from build123d import *

# Parameters (mm, degrees)
SKETCH_1_W          = 82
SKETCH_1_H          = 66
SKETCH_1_R          = 1.6
SKETCH_1_R_2        = 1.35
EXTRUDE_1_DEPTH     = 2
FILLET_1_R          = 3
CUT_EXTRUDE_1_DEPTH = 10
SKETCH_3_R          = 27.5
SKETCH_3_R_2        = 24.5
SKETCH_3_W          = 10
SKETCH_3_H          = 3
EXTRUDE_1_2_DEPTH   = 2
SKETCH_4_R          = 1.1
CUT_EXTRUDE_2_DEPTH = 2
FILLET_2_R          = 1


with BuildPart() as part:
    # 草图1 → Extrude 1 (new body)
    with BuildSketch(Plane(origin=(0, 0, 0), x_dir=(1, 0, 0), z_dir=(0, 1, 0))):
        Rectangle(SKETCH_1_W, SKETCH_1_H)
        with Locations(Location((10, -30, 0), (0, 0, 270))):
            Circle(SKETCH_1_R, mode=Mode.SUBTRACT)
        with Locations(Location((-10, -30, 0), (0, 0, 270))):
            Circle(SKETCH_1_R, mode=Mode.SUBTRACT)
        with Locations(Location((-10, 30, 0), (0, 0, 270))):
            Circle(SKETCH_1_R, mode=Mode.SUBTRACT)
        with Locations(Location((10, 30, 0), (0, 0, 270))):
            Circle(SKETCH_1_R, mode=Mode.SUBTRACT)
        with Locations(Location((36, -27, 0), (0, 0, 270))):
            Circle(SKETCH_1_R_2, mode=Mode.SUBTRACT)
        with Locations(Location((36, 27, 0), (0, 0, 270))):
            Circle(SKETCH_1_R_2, mode=Mode.SUBTRACT)
        with Locations(Location((-36, 27, 0), (0, 0, 270))):
            Circle(SKETCH_1_R_2, mode=Mode.SUBTRACT)
        with Locations(Location((-36, -27, 0), (0, 0, 270))):
            Circle(SKETCH_1_R_2, mode=Mode.SUBTRACT)
    extrude(amount=EXTRUDE_1_DEPTH)

    # 圆角1
    fillet_1_edges = [part.edges().sort_by_distance(p)[0] for p in [
        (41, 1, 33),
        (-41, 1, 33),
        (-41, 1, -33),
        (41, 1, -33),
    ]]
    fillet(fillet_1_edges, radius=FILLET_1_R)

    # 草图2 → 切除-拉伸1 (cut)
    with BuildSketch(Plane(origin=(0, 2, 0), x_dir=(1, 0, 0), z_dir=(0, 1, 0))):
        with BuildLine():
            Line((32.385791926, 26), (-32.385791926, 26))
            ThreePointArc((-32.385791926, 26), (-33.729262234, 24.015665903), (-36, 23.25))
            Line((-36, 23.25), (-36, -23.25))
            ThreePointArc((-36, -23.25), (-33.729262234, -24.015665903), (-32.385791926, -26))
            Line((-32.385791926, -26), (32.385791926, -26))
            ThreePointArc((32.385791926, -26), (33.729262234, -24.015665903), (36, -23.25))
            Line((36, -23.25), (36, 23.25))
            ThreePointArc((36, 23.25), (33.729262234, 24.015665903), (32.385791926, 26))
        make_face()
    extrude(amount=-CUT_EXTRUDE_1_DEPTH, mode=Mode.SUBTRACT)

    # 草图3 → Extrude 1 2 (add)
    # profile 1 of 5: a face of its own
    with BuildSketch(Plane(origin=(0, 2, 0), x_dir=(1, 0, 0), z_dir=(0, 1, 0))):
        Circle(SKETCH_3_R)
        Circle(SKETCH_3_R_2, mode=Mode.SUBTRACT)
    # profile 2 of 5: a face of its own
    with BuildSketch(Plane(origin=(0, 2, 0), x_dir=(1, 0, 0), z_dir=(0, 1, 0))):
        Polygon((36.9, -25.8), (-35.1, 28.2), (-36.9, 25.8), (35.1, -28.2), align=None)
    # profile 3 of 5: a face of its own
    with BuildSketch(Plane(origin=(0, 2, 0), x_dir=(1, 0, 0), z_dir=(0, 1, 0))):
        Polygon((-35.1, -28.2), (36.9, 25.8), (35.1, 28.2), (-36.9, -25.8), align=None)
    # profile 4 of 5: a face of its own
    with BuildSketch(Plane(origin=(0, 2, 0), x_dir=(1, 0, 0), z_dir=(0, 1, 0))):
        with Locations((-31, 0)):
            Rectangle(SKETCH_3_W, SKETCH_3_H)
    # profile 5 of 5: a face of its own
    with BuildSketch(Plane(origin=(0, 2, 0), x_dir=(1, 0, 0), z_dir=(0, 1, 0))):
        with Locations((31, 0)):
            Rectangle(SKETCH_3_W, SKETCH_3_H)
    extrude(amount=-EXTRUDE_1_2_DEPTH)

    # 草图4 → 切除-拉伸2 (cut)
    with BuildSketch(Plane(origin=(0, 2, 0), x_dir=(1, 0, 0), z_dir=(0, 1, 0))):
        with Locations((36, 27)):
            Circle(SKETCH_4_R)
        with Locations((-36, 27)):
            Circle(SKETCH_4_R)
        with Locations((-36, -27)):
            Circle(SKETCH_4_R)
        with Locations((36, -27)):
            Circle(SKETCH_4_R)
    extrude(amount=-CUT_EXTRUDE_2_DEPTH, mode=Mode.SUBTRACT)

    # 圆角2
    fillet_2_edges = [part.edges().sort_by_distance(p)[0] for p in [
        (-34.150454583, 1, 23.737840937),
        (-8.958236434, 1, 26),
        (8.958236434, 1, 26),
        (-32.166666667, 1, 26),
        (32.166666667, 1, 26),
        (34.150454583, 1, 23.737840937),
        (34.150454583, 1, -23.737840937),
        (-8.958236434, 1, -26),
        (8.958236434, 1, -26),
        (32.166666667, 1, -26),
        (-32.166666667, 1, -26),
        (-34.150454583, 1, -23.737840937),
        (21.067248348, 1, 17.675436261),
        (-21.067248348, 1, 17.675436261),
        (0, 1, -1.875),
        (-18.663230817, 1, -15.872423113),
        (20.463230817, 1, 13.472423113),
        (0, 1, 1.875),
        (-22.867248348, 1, -15.275436261),
        (-22.867248348, 1, 15.275436261),
        (-27.459060435, 1, 1.5),
        (-36, 1, 1.5),
        (-27.459060435, 1, -1.5),
        (-36, 1, -1.5),
        (-20.463230817, 1, -13.472423113),
        (-20.463230817, 1, 13.472423113),
        (18.663230817, 1, 15.872423113),
        (-2.5, 1, 0),
        (-18.663230817, 1, 15.872423113),
        (2.5, 1, 0),
        (20.463230817, 1, -13.472423113),
        (21.067248348, 1, -17.675436261),
        (-21.067248348, 1, -17.675436261),
        (18.663230817, 1, -15.872423113),
        (22.867248348, 1, -15.275436261),
        (36, 1, 1.5),
        (27.459060435, 1, -1.5),
        (36, 1, -1.5),
        (22.867248348, 1, 15.275436261),
        (27.459060435, 1, 1.5),
        (-36, 1, -23.25),
        (36, 1, -23.25),
        (36, 1, 23.25),
        (-36, 1, 23.25),
    ]]
    fillet(fillet_2_edges, radius=FILLET_2_R)


solid = part.part
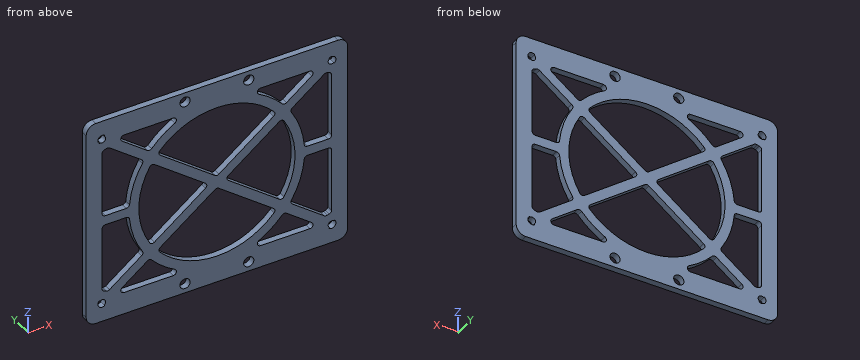
The listing builds one solid part. Answer for the finished solid, in the listing's coordinates (mm). Coordinates: 2 decimals unless noted, no trailing zeros. Order: outer loops, then holes, each group sorted by start corner. A loop starts at its lowest first (then second) coordinate and runs counter-clockwise, first axis right, second up. Notation, with made-up numbers: M -20,87 L -15,87 A35 ccw -15,119 Z; hole C 9,8 d4. An arc over 180 degrees is marked long. Use CSV: the item, a comma, the result in double quotes.
Q1. Section C-C (y = 1.65) is taken. Give the number of separate pieces and of enclosed holes in the cut face, then the cut area to 3 significant figures.
Here are the results:
separate pieces,"1"
enclosed holes,"20"
area,"2,620 mm2"
Q2. Straight lines are drawn through the part: L1, parallel to X at y = 1.35, z = -30; L2, parallel to X at y = 1.5, z = -27; L3, parallel to Z at x = 15, y = 0.2 (3 decimals). For each, find the intervals that lie inside material, in ascending order.
Here are the results:
L1,"-41 to -11.6, -8.4 to 8.4, 11.6 to 41"
L2,"-41 to -37.35, -34.9 to 34.9, 37.35 to 41"
L3,"-33 to -26, -23.049 to -19.371, -13.125 to -9.375, 9.375 to 13.125, 19.371 to 23.049, 26 to 33"
Q3. Given pin 1 Ø2.5 at (x, z) = (-10, -30) entering from +Y, flat-ended and moving along its own axis, determine where the tip first touches the part or whether it passes through.
Here are the results:
pin 1,"through"
Q4. Section A-A (x = -10) is taken. Determine the outline of the cut face in (y, z) (3 decimals), then the cut area to 3 significant figures.
Here are the results:
outline,"M 0,-33 L 2,-33 L 2,-31.6 L 0,-31.6 Z; M 0,-28.4 L 2,-28.4 L 2,-22.366 L 0,-22.366 Z; M 0,-9.375 L 2,-9.375 L 2,-5.625 L 0,-5.625 Z; M 0,5.625 L 2,5.625 L 2,9.375 L 0,9.375 Z; M 0,22.366 L 2,22.366 L 2,28.4 L 0,28.4 Z; M 0,31.6 L 2,31.6 L 2,33 L 0,33 Z"
area,"44.7 mm2"
Q5. Section B-B (z = 21) is taken. Determine the outline of the cut face in (x, y).
Here are the results:
outline,"M -41,0 L -36,0 L -36,2 L -41,2 Z; M -30.5,0 L -25.5,0 L -25.5,2 L -30.5,2 Z; M -17.76,0 L -12.62,0 L -12.62,2 L -17.76,2 Z; M 12.62,0 L 17.76,0 L 17.76,2 L 12.62,2 Z; M 25.5,0 L 30.5,0 L 30.5,2 L 25.5,2 Z; M 36,0 L 41,0 L 41,2 L 36,2 Z"
